Source: CAD feature listing. Evaluate the final solid. Frame: model axes, mm. Coordinates: 2 decimals unless noted, no trailing zeros. Order: outer loops, then holes, each group sorted by start corner. A loop starts at its lowest first (then second) coordinate and runs counter-clockwise, first axis right, second up.
Item 1: Section B-B on z = -57. Return the cut outline in (x, y) (3 decimals).
Item 2: Section A-A on x = 7.5. Return the cut outline in (y, z) (3 decimals), then the cut area to 3 significant figures.
Item 3: Ray query, line 1 (Y direction, x = 6.5, z = 55) (3 decimals); line 2 (Y direction, x = 17.95, z = -50.8); line 3 (X direction, y = 4, z = 67) (3 decimals). Return the intervals inside material, ascending.
from build123d import *

# Parameters (mm, degrees)
BOSS_EXTRUDE1_DEPTH      = 317.499999
BOSS_EXTRUDE1_DEPTH_BACK = 317.499999
SKETCH3_W                = 38.1
SKETCH3_H                = 25.4
SKETCH3_W_2              = 31.75
SKETCH3_H_2              = 19.05
MOUNTING_HOLES_D         = 4.9784
RIO_HOLES_D              = 4.9784
F_10_CLEARANCE_HOLE1_D   = 4.9784


with BuildPart() as part:
    # Sketch3 → Boss-Extrude1 (new, two sides: drawn at the far end of the back side and taken through both)
    with BuildSketch(Plane.XY.offset(-BOSS_EXTRUDE1_DEPTH_BACK)):
        Rectangle(SKETCH3_W, SKETCH3_H)
        Rectangle(SKETCH3_W_2, SKETCH3_H_2, mode=Mode.SUBTRACT)
    extrude(amount=BOSS_EXTRUDE1_DEPTH + BOSS_EXTRUDE1_DEPTH_BACK)

    # Mounting Holes (through all)
    with Locations(Plane.ZY.offset(19.05)):
        with Locations((279.400000508, 0), (304.800000508, 0), (-76.2, 0)):
            Hole(MOUNTING_HOLES_D / 2)

    # Rio Holes (through all)
    with Locations(Plane.ZY.offset(19.05)):
        with Locations((-50.8, 0), (50.8, 0)):
            Hole(RIO_HOLES_D / 2)

    # SurfaceCut1
    split(bisect_by=Plane(origin=(0, 0, -88.899999492), x_dir=(-1, 0, 0), z_dir=(0, 0, -1)), keep=Keep.BOTTOM)

    # #10 Clearance Hole1 (through all)
    with Locations(Plane(origin=(19.05, 0, 0), x_dir=(0, 0, -1), z_dir=(1, 0, 0))):
        with Locations((-252.857000508, -5.03e-07), (-227.457000508, -5.03e-07), (-99.187000508, -1.231595708), (-124.587000508, -1.231595708)):
            Hole(F_10_CLEARANCE_HOLE1_D / 2)


solid = part.part
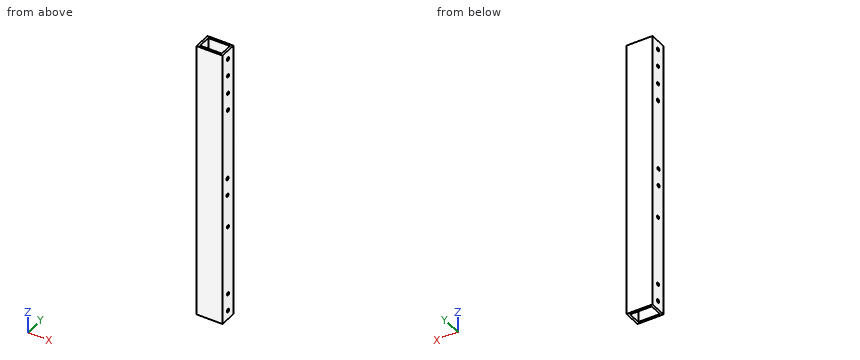
Answer list:
1. outline: (-19.05, -12.7) - (19.05, -12.7) - (19.05, 12.7) - (-19.05, 12.7) - close; hole (-15.875, -9.525) - (15.875, -9.525) - (15.875, 9.525) - (-15.875, 9.525) - close
2. outline: (-12.7, -88.9) - (-9.525, -88.9) - (-9.525, 317.5) - (-12.7, 317.5) - close; (9.525, -88.9) - (12.7, -88.9) - (12.7, 317.5) - (9.525, 317.5) - close
2. area: 2,580 mm2
3. line 1: y = -12.7 to -9.525, 9.525 to 12.7
3. line 2: y = -12.7 to -2.49, 2.49 to 12.7
3. line 3: x = -19.05 to -15.875, 15.875 to 19.05
